```python
from build123d import *

# Parameters (mm, degrees)
F1_DEPTH = 5
F2_W     = 35.7
F2_H     = 45.25
F4_W     = 44
F4_H     = 45.25
F6_DEPTH = 1.5
F8_DEPTH = 2.5
F9_R     = 1


# Not quite as in the source:
# - a pattern or mirror of a feature is missing from the dataset's text; its kind, count and spacing are read off the source's solid


with BuildPart() as f1:
    # F0 (on Top) → F1 (new body)
    with BuildSketch(Plane.XY):
        with BuildLine():
            Line((-15.85, -31.425), (15.85, -31.425))
            ThreePointArc((15.85, -31.425), (17.2642135624, -30.8392135624), (17.85, -29.425))
            Line((17.85, -29.425), (17.85, 29.425))
            ThreePointArc((17.85, 29.425), (17.2642135624, 30.8392135624), (15.85, 31.425))
            Line((15.85, 31.425), (-15.85, 31.425))
            ThreePointArc((-15.85, 31.425), (-17.2642135624, 30.8392135624), (-17.85, 29.425))
            Line((-17.85, 29.425), (-17.85, -29.425))
            ThreePointArc((-17.85, -29.425), (-17.2642135624, -30.8392135624), (-15.85, -31.425))
        make_face()
    extrude(amount=-F1_DEPTH)

    # F2 (on face) → F5 section 0
    with BuildSketch(Plane(origin=(0, 0, -5), x_dir=(1, 0, 0), z_dir=(0, 0, -1))):
        Rectangle(F2_W, F2_H)
    # F4 (on offset) → F5 section 1
    with BuildSketch(Plane(origin=(0, 0, -11.85), x_dir=(1, 0, 0), z_dir=(0, 0, -1))):
        Rectangle(F4_W, F4_H)
    loft()

    # F4 (on offset) → F6 (join)
    with BuildSketch(Plane(origin=(0, 0, -11.85), x_dir=(1, 0, 0), z_dir=(0, 0, -1))):
        Rectangle(F4_W, F4_H)
    extrude(amount=F6_DEPTH)

    # F7 (on face) → F8 (cut)
    with BuildSketch(Plane.XZ.offset(22.625)):
        Polygon((5.9, -5), (0, -5), (-5.9, -5), (-5.9, -9.3), (0, -9.3), (5.9, -9.3), align=None)
        Polygon((-7.6, -9.3), (-7.6, -5), (-17.85, -5), (-20.4551094891, -9.3), align=None)
        Polygon((17.85, -5), (7.6, -5), (7.6, -9.3), (20.4551094891, -9.3), align=None)
    f8 = extrude(amount=-F8_DEPTH, mode=Mode.SUBTRACT)

    # F8_copies: F8 across plane
    add(f8.mirror(Plane.ZX), mode=Mode.SUBTRACT)

    # F9
    f9_edges = [f1.edges().sort_by_distance(p)[0] for p in [
        (-14.027555, -20.125, -9.3),
        (0, -20.125, -9.3),
        (14.027555, -20.125, -9.3),
        (14.027555, 20.125, -9.3),
        (0, 20.125, -9.3),
        (-14.027555, 20.125, -9.3),
    ]]
    fillet(f9_edges, radius=F9_R)


solid = f1.part
```
Model file for the job. Use its own axes, mm. A direction names the side the tool comes from. Give positions to 0.01 mm unless a question says otherwise; leave off trailing zeros. Order: outer loops, then holes, each group sorted by start corner. A loop starts at its lowest first (then second) coordinate and runs counter-clockwise, first axis right, second up.
1) Mould opens along Z. For faces 1 (the flat face through (19.95, 0.32, -8.47)), 2 (the flat face through (22, 0, -13)), 3 (the flat face through (0, 20.125, -7)), 4 (the flat face through (14, 20.125, -7)) say: +Z half, -Z half, draft (parallel to the pull), parting line (faces both ways), or undercut.
2) Saw through at B-B, the plane z = -1.5. Write the cut outline in (x, y) (3 decimals), then the cut area to 3 significant figures.
3) Saw through at A-A, the plane y = -22. Write the cut outline in (x, z), then the cut area to 3 significant figures.
4) Wall check: probe 1 along X at (y, z) = (27, -2.5); probe 2 along Y at (x, z) = (-15.5, -10.25) (3 decimals); probe 3 along Z at (x, y) = (-7.5, 26.5). Give the ranges that are in metal, low to high.
5) Pin check, flat tips, straight feed: pin 1 (3 mm diameter, centred on y = -21.5, z = -7, fed in from +X); pin 2 (1.2 mm diameter, centred on y = 21.5, z = -7, fed in from -X); pin 3 (3 mm diameter, centred on y = 13, z = -4, fed in from -X). Stop position of each tip, or through.
6) 3-axis set-ups, long thin cutter, end or side, ignore diameter. For faces 5 (the flat face through (17.85, 0, -2)), 6 (the flat face through (7.6, -21, -7)), 7 (the flat face through (0, 22, -9.3)), 8 (the flat face through (-7.6, 21, -7)), 9 (the flat face through (-7.6, -21, -7)): which of +Z, -Z, +X, -X, +Y, -Y reach the whole face in a straight line?
7) Saw through at D-D, the plane z = -5.75. Write the cut outline in (x, y) (3 decimals), then the cut area to 3 significant figures.
8) Saw through at C-C, the plane x = -3.5. Write the cut outline in (y, z) (3 decimals).
Computed:
1. face 1: +Z half
1. face 2: draft
1. face 3: undercut
1. face 4: undercut
2. outline: (-17.85, -29.425) arc R2 ccw to (-15.85, -31.425) - (15.85, -31.425) arc R2 ccw to (17.85, -29.425) - (17.85, 29.425) arc R2 ccw to (15.85, 31.425) - (-15.85, 31.425) arc R2 ccw to (-17.85, 29.425) - close
2. area: 2,240 mm2
3. outline: (-22, -13.35) - (22, -13.35) - (22, -11.85) - (20.46, -9.3) - (7.6, -9.3) - (7.6, -5) - (17.85, -5) - (17.85, 0) - (-17.85, 0) - (-17.85, -5) - (-7.6, -5) - (-7.6, -9.3) - (-20.46, -9.3) - (-22, -11.85) - close; hole (-5.9, -9.3) - (5.9, -9.3) - (5.9, -5) - (-5.9, -5) - close
3. area: 367 mm2
4. probe 1: x = -17.85 to 17.85
4. probe 2: y = -22.625 to 22.625
4. probe 3: z = -5 to 0
5. pin 1: stops at x = 19.42
5. pin 2: stops at x = -7.6
5. pin 3: stops at x = -18.15
6. face 5: +Z, +X, +Y, -Y
6. face 6: +X, -Y
6. face 7: +Y
6. face 8: -X, +Y
6. face 9: -X, -Y
7. outline: (-18.304, -20.125) - (-7.6, -20.125) - (-7.6, -22.625) - (-5.9, -22.625) - (-5.9, -20.125) - (5.9, -20.125) - (5.9, -22.625) - (7.6, -22.625) - (7.6, -20.125) - (18.304, -20.125) - (18.304, 20.125) - (7.6, 20.125) - (7.6, 22.625) - (5.9, 22.625) - (5.9, 20.125) - (-5.9, 20.125) - (-5.9, 22.625) - (-7.6, 22.625) - (-7.6, 20.125) - (-18.304, 20.125) - close
7. area: 1,490 mm2
8. outline: (-31.425, -5) - (-20.125, -5) - (-20.125, -8.3) arc R1 cw to (-21.125, -9.3) - (-22.625, -9.3) - (-22.625, -13.35) - (22.625, -13.35) - (22.625, -9.3) - (21.125, -9.3) arc R1 cw to (20.125, -8.3) - (20.125, -5) - (31.425, -5) - (31.425, 0) - (-31.425, 0) - close
